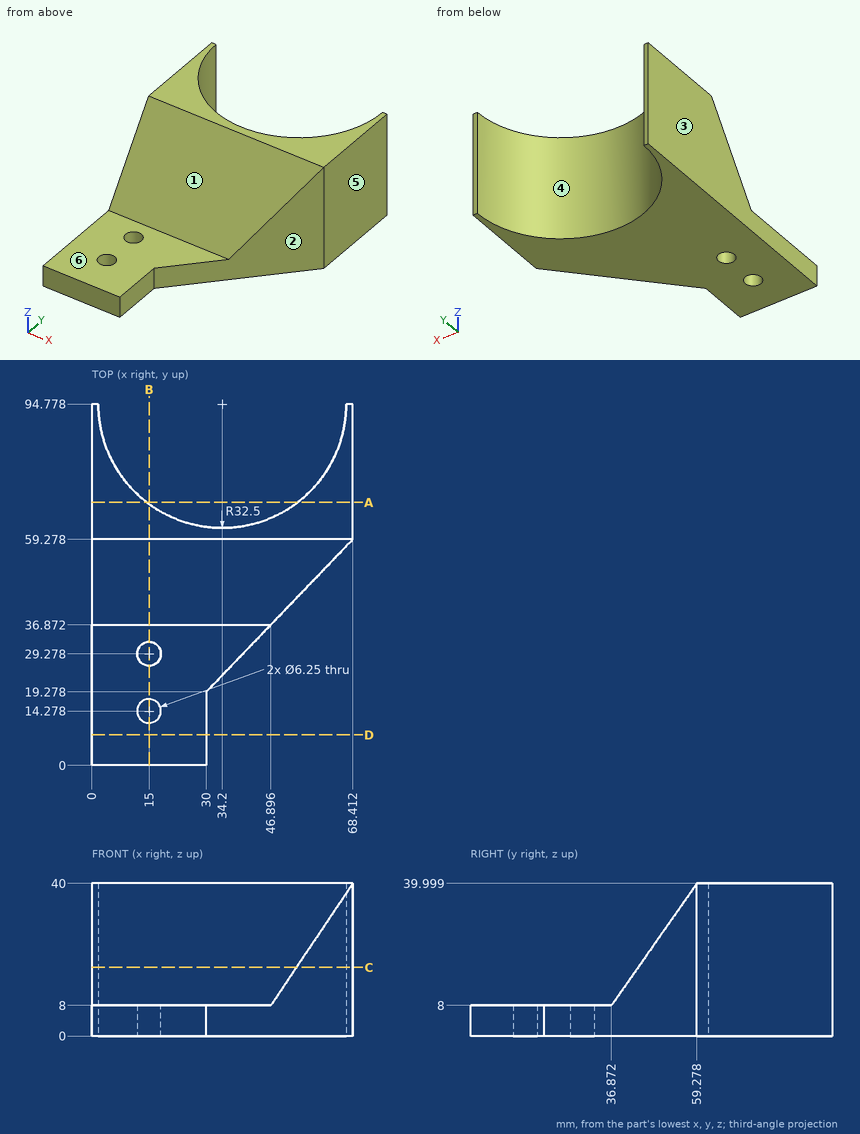
Design review of the part shown in the three views and the two pictorial views. Dimensions are in mm from the part's minimum x, y and z. A direction names the side the tool comes from. Round coordinates to 2 decimals unless told otherwise and drop trailing zeros. Write each loop counter-clockwise with the first axis right and the second up, starting at its lowest first coordinate (ties: lowest second). Pieces come first, ordered by that corner, then holes. Notation, with made-up numbers: M 4.5,56.5 L 42.5,56.5 A3 cw 42.5,60.5 Z; hole C 18,-23 d10. An arc over 180 degrees is marked long. One line per item, written item: value. Start each with the question number.
1. Draft analysis for pull direction X (two halves, no side actions). For the marked faces 1, 2, 3 and 4, state which applies: pulls with the +X half, pulls with the -X half, needs draft (parallel to the pull), parting line crosses it, or undercut.
2. Take a section at D-D on y = 8. State the section outline as (x, z) points, then the cut area to 3 significant figures.
3. To check wall thickness, follow probe 1 along Y at (x, z) = (15, 3) (1 decimal); probe 2 along X at (y, z) = (14, 6.5); probe 3 along Z at (x, y) = (21.5, 26). State the ranges of each line that lie inside material, in increasing order. Write a range as from..to.
4. Take a section at B-B on x = 15. State how many separate pieces and enclosed holes the cut face has, then the cut area to 3 significant figures.
5. Take a section at A-A on y = 69. State the section outline as (x, z) points.
6. For the marked faces 5 and 6, list the 3-axis set-ups (+Z, -Z, +X, -X, +Y, -Y) from which the entire face can be reached by the end or side of a thin tool; tool diameter is ignored.
7. Take a section at C-C on z = 18. State the section outline as (x, y) points (1 decimal), then the cut area to 3 significant figures.
8. Clearance check with flat-ended pins moving along their axes: P1, Ø8, axis at y = 66, z = 8.5, coming from the -X side; P2, Ø6, axis at x = 56.5, z = 14.5, coming from the +Y side; P3, Ø2.5, axis at y = 6.5, z = 5, coming from the +X side; P4, Ø5, axis at x = 19.5, z = 29, coming from the +Y side. State where each tip first meets the part, or that it passes through.
Computed:
1. face 1: needs draft
1. face 2: pulls with the +X half
1. face 3: pulls with the -X half
1. face 4: undercut
2. outline: M 0,0 L 30,0 L 30,8 L 0,8 Z
2. area: 240 mm²
3. probe 1: y = 0..11.2, 17.4..26.2, 32.4..68.6
3. probe 2: x = 0..11.89, 18.11..30
3. probe 3: z = 0..8
4. separate pieces: 3
4. enclosed holes: 0
4. area: 1,100 mm²
5. outline: M 0,0 L 14.41,0 L 14.41,40 L 0,40 Z; M 53.99,0 L 68.41,0 L 68.41,40 L 53.99,40 Z
6. face 5: +Z, -Z, +X, +Y, -Y
6. face 6: +Z, +X, -X, -Y
7. outline: M 0,43.9 L 53.6,43.9 L 68.4,59.3 L 68.4,94.8 L 66.7,94.8 A32.5 cw 1.7,94.8 L 0,94.8 Z
7. area: 1,710 mm²
8. P1: stops at x = 0
8. P2: stops at y = 74.38
8. P3: stops at x = 30
8. P4: stops at y = 67.2
